```python
from build123d import *

# Parameters (mm, degrees)
F0_W     = 8
F0_H     = 1
F0_W_2   = 7.7403839678
F0_W_3   = 13
F1_DEPTH = 7
F2_R     = 3
F3_R     = 2


with BuildPart() as f1:
    # F0 (on Top) → F1 (new body)
    with BuildSketch(Plane.XY):
        with BuildLine():
            Line((-40.8660421073, 35.5213209987), (-62.8660421073, 35.5213209987))
            ThreePointArc((-62.8660421073, 35.5213209987), (-65.6944692321, 34.3497481234), (-66.8660421073, 31.5213209987))
            Line((-66.8660421073, 31.5213209987), (-66.8660421073, 5.6138705388))
            Line((-66.8660421073, 5.6138705388), (-65.8120451986, 5.6138705388))
            ThreePointArc((-65.8120451986, 5.6138705388), (-65.5673840665, 5.5125285796), (-65.4660421073, 5.2678674475))
            Line((-65.4660421073, 5.2678674475), (-65.4660421073, -2.04012637))
            ThreePointArc((-65.4660421073, -2.04012637), (-65.5673840665, -2.2847875021), (-65.8120451986, -2.3861294612))
            Line((-65.8120451986, -2.3861294612), (-66.8660421073, -2.3861294612))
            Line((-66.8660421073, -2.3861294612), (-66.8660421073, -33.4786790013))
            ThreePointArc((-66.8660421073, -33.4786790013), (-65.6944692321, -36.3071061261), (-62.8660421073, -37.4786790013))
            Line((-62.8660421073, -37.4786790013), (67.1339578927, -37.4786790013))
            ThreePointArc((67.1339578927, -37.4786790013), (69.9623850174, -36.3071061261), (71.1339578927, -33.4786790013))
            Line((71.1339578927, -33.4786790013), (71.1339578927, 31.5213209987))
            ThreePointArc((71.1339578927, 31.5213209987), (69.9623850174, 34.3497481234), (67.1339578927, 35.5213209987))
            Line((67.1339578927, 35.5213209987), (52.1339578927, 35.5213209987))
            Line((52.1339578927, 35.5213209987), (39.1339578927, 35.5213209987))
            Line((39.1339578927, 35.5213209987), (27.1339578927, 35.5213209987))
            Line((27.1339578927, 35.5213209987), (19.3935739249, 35.5213209987))
            Line((19.3935739249, 35.5213209987), (-32.8660421073, 35.5213209987))
            Line((-32.8660421073, 35.5213209987), (-40.8660421073, 35.5213209987))
        make_face()
        with Locations((-36.8660421073, 36.0213209987)):
            Rectangle(F0_W, F0_H)
        with BuildLine():
            Line((-65.8120451986, 5.6138705388), (-66.8660421073, 5.6138705388))
            Line((-66.8660421073, 5.6138705388), (-66.8660421073, -2.3861294612))
            Line((-66.8660421073, -2.3861294612), (-65.8120451986, -2.3861294612))
            ThreePointArc((-65.8120451986, -2.3861294612), (-65.5673840665, -2.2847875021), (-65.4660421073, -2.04012637))
            Line((-65.4660421073, -2.04012637), (-65.4660421073, 5.2678674475))
            ThreePointArc((-65.4660421073, 5.2678674475), (-65.5673840665, 5.5125285796), (-65.8120451986, 5.6138705388))
        make_face()
        with Locations((23.2637659088, 36.0213209987)):
            Rectangle(F0_W_2, F0_H)
        with Locations((45.6339578927, 36.0213209987)):
            Rectangle(F0_W_3, F0_H)
    extrude(amount=F1_DEPTH)

    # F2
    f2_edges = [f1.edges().sort_by_distance(p)[0] for p in [
        (2.133958, -37.478679, 7),
    ]]
    fillet(f2_edges, radius=F2_R)

    # F3
    f3_edges = [f1.edges().sort_by_distance(p)[0] for p in [
        (2.133958, -37.478679, 0),
        (-6.736234, 35.521321, 0),
        (33.133958, 35.521321, 0),
    ]]
    fillet(f3_edges, radius=F3_R)


solid = f1.part
```
Geometry check sheet. Reference: the model listing, model coordinates, mm. A direction names the side the tool comes from. Give positions to 0.01 mm unless a question says otherwise; leave off trailing zeros. Write each loop counter-clockwise with the first axis right and the second up, starting at its lowest first coordinate (ties: lowest second). Pieces come first, ordered by that corner, then holes.
1) Release check for a two-part mould opening along X. For faces 4 (the cylindrical face through (-66.01, -1.43, 6.1)), 5 (the flat face through (33, 35.521, 4)), 6 (the cylindrical face through (69.93, -36.34, 2.99)) record: pulls with the +X half, pulls with the -X half, needs draft (parallel to the pull), parting line crosses it, or undercut.
2) Section check B-B, the plane x = 28.5. Record the boundary of the cut face in (y, z), and give its area (3 significant figures).
3) Gauge pin test, flat ends, axial feed: pin 1 (0.6 mm diameter, centred on x = -54.5, z = 3, fed in from +Y); pin 2 (2.5 mm diameter, centred on y = 34.5, z = 2.5, fed in from +X); pin 3 (0.9 mm diameter, centred on y = 35, z = 4.5, fed in from -X) (3 decimals). Record the tip position at first contact, or that the pin passes through.
4) Section check A-A, the plane x = -45. Record the boundary of the cut face in (y, z), and give its area (3 significant figures).
5) Access from +Z, -Z, +X, -X, +Y, -Y to the whole of each face (thin tool, end or side, straight path). Record for faces 1 (the flat face through (-6, 35.521, 4)), 2 (the flat face through (39.134, 36, 3)), 3 (the flat face through (-37, 36.521, 3)).
6) Material ranges on L1, parallel to Y at x = -60.5, z = 3.75; L2, parallel to Z at x = 60.5, y = 33.5; L3, parallel to Y at x = -32, z = 1, recorded low to high.
Computed:
1. face 4: pulls with the -X half
1. face 5: undercut
1. face 6: pulls with the +X half
2. outline: (-37.48, 2) arc R2 ccw to (-35.48, 0) - (33.52, 0) arc R2 ccw to (35.52, 2) - (35.52, 7) - (-34.48, 7) arc R3 ccw to (-37.48, 4) - close
2. area: 507 mm2
3. pin 1: stops at y = 35.52
3. pin 2: stops at x = 70.74
3. pin 3: stops at x = -65.425
4. outline: (-37.48, 2) arc R2 ccw to (-35.48, 0) - (33.52, 0) arc R2 ccw to (35.52, 2) - (35.52, 4) arc R3 ccw to (32.52, 7) - (-34.48, 7) arc R3 ccw to (-37.48, 4) - close
4. area: 505 mm2
5. face 1: +Z, -Z, +Y
5. face 2: -Z, +Y
5. face 3: +Z, -Z, +X, -X, +Y
6. L1: y = -37.48 to 35.52
6. L2: z = 0 to 6.84
6. L3: y = -37.21 to 35.25
